Model file for the job. Use its own axes, mm. A direction names the side the tool comes from. Give positions to 0.01 mm unless a question says otherwise; leave off trailing zeros. Loops run counter-clockwise (first coordinate to the right, second up) from the corner with the lowest first, then second, coordinate; pieces in that order, holes last. Notation, with made-up numbers: (-27.75, -25) - (7.25, -25) arc R14 ccw to (7.25, -2) - close; hole circle Ø1 at (15, -14). An arc over 180 degrees is marked (long way). Use a Markdown table: item, result.
from build123d import *

# Parameters (mm, degrees)
F4_DEPTH = 19.3304


with BuildPart() as f1:
    # F0 (on Right) → F1 (revolve)
    with BuildSketch(Plane.YZ):
        with BuildLine():
            Line((123.1392, 241.1603), (116.679401, 252.349))
            Line((116.679401, 252.349), (104.4702, 252.349))
            Line((104.4702, 252.349), (104.4702, 287.274))
            Line((104.4702, 287.274), (75.8952, 287.274))
            Line((75.8952, 287.274), (75.8952, 255.524))
            Line((75.8952, 255.524), (25.4, 255.524))
            Line((25.4, 255.524), (25.4, 245.0338))
            Line((25.4, 245.0338), (0, 125.476))
            Line((0, 125.476), (0, 0))
            Line((0, 0), (50.8, 0))
            Line((50.8, 0), (50.8, 221.123768))
            ThreePointArc((50.8, 221.123768), (51.283365, 223.553808), (52.659872, 225.613896))
            Line((52.659872, 225.613896), (62.430488, 235.384512))
            ThreePointArc((62.430488, 235.384512), (70.670841, 240.89054), (80.391, 242.824))
            Line((80.391, 242.824), (98.440942, 242.824))
            Line((98.440942, 242.824), (110.3376, 239.6363))
            Line((110.3376, 239.6363), (123.1392, 239.6363))
            Line((123.1392, 239.6363), (123.1392, 241.1603))
        make_face()
    revolve(axis=Axis((0, 61.5696, 0), (0, 1, 0)))

    # F3 (on offset) → F4 (cut, through all)
    with BuildSketch(Plane(origin=(0, 19.3294, 0), x_dir=(-1, 0, 0), z_dir=(0, 1, 0))):
        with BuildLine():
            Line((-77.1779, 197.1167), (77.1779, 197.1167))
            ThreePointArc((77.1779, 197.1167), (87.122, 207.0608), (77.1779, 217.0049))
            Line((77.1779, 217.0049), (-77.1779, 217.0049))
            ThreePointArc((-77.1779, 217.0049), (-87.122, 207.0608), (-77.1779, 197.1167))
        make_face()
    extrude(amount=-F4_DEPTH, mode=Mode.SUBTRACT)


solid = f1.part
(1) Slice it at B-B, the plane y = 40.5. Write the cut outline in (x, z), plus the area to 3 significant figures.
Computed:
| item | result |
|---|---|
| outline | circle Ø511.05 at (0, 0) |
| area | 205,000 mm² |
(2) Pin check, flat tips, straight feed: P1, Ø8, axis at x = -78.5, z = -177.5, coming from the +Y side; P2, Ø5, axis at y = 32.5, z = 132, coming from the +X side; P3, Ø1, axis at y = 78.5, z = -4, coming from the -X side. Stop position of each tip, or through.
Computed:
| item | result |
|---|---|
| P1 | y = 50.8 |
| P2 | x = 220.28 |
| P3 | x = -287.25 |
(3) 3-axis set-ups, long thin cutter, end or side, ignore diameter. For faces 4 (the cylindrical face through (72.94, 89.54, 231.61)), 5 (the cylindrical face through (253.35, 50.29, -33.26)), 6 (the flat face through (3, 50.8, 3)): which of +Z, -Z, +X, -X, +Y, -Y reach the whole face in a straight line?
Computed:
| item | result |
|---|---|
| face 4 | none |
| face 5 | -Y |
| face 6 | +Y |
(4) Mould opens along X. For faces 1 (the conical face through (-220.846, 53.271, -49.041)), 2 (the flat face through (-254, 104.47, 1)), 3 (the cylindrical face through (-246.35, 110.49, -54.7)) say: pulls with the +X half, pulls with the -X half, needs draft (parallel to the pull), parting line crosses it, or undercut.
Computed:
| item | result |
|---|---|
| face 1 | undercut |
| face 2 | needs draft |
| face 3 | parting line crosses it |
(5) Drill centre lines: probe 1 along X at (y, z) = (90.5, 0); probe 2 along X at (y, z) = (116.5, 0); probe 3 along Y at (x, z) = (3, 114.5). Where is each one in solid material? Low to high. Write a range as [from, to].
Computed:
| item | result |
|---|---|
| probe 1 | [-287.27, -242.82], [242.82, 287.27] |
| probe 2 | [-252.35, -239.64], [239.64, 252.35] |
| probe 3 | [0, 50.8] |
